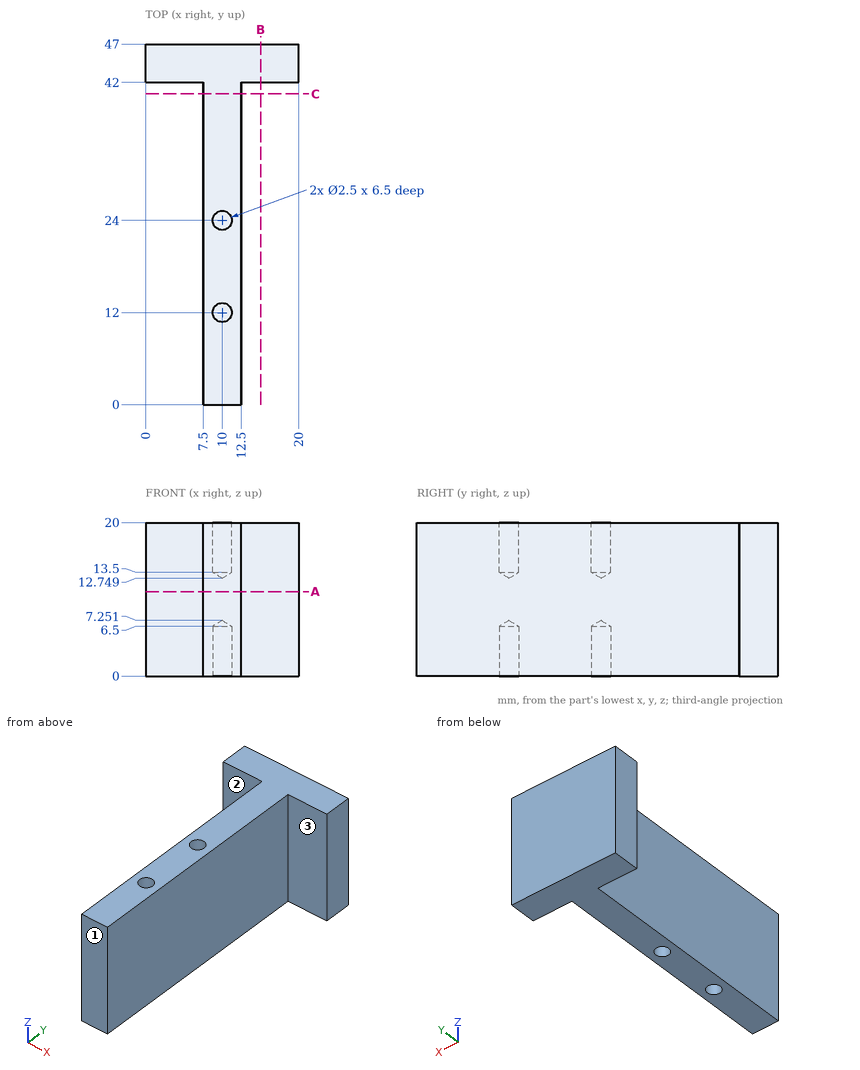
Verification items for this drawing (mm, ordinates from the low corner). A direction names the side the tool comes from. Coordinates: 2 decimals unless noted, no trailing zeros. Loops run counter-clockwise (first coordinate to the right, second up) from the corner with the lowest first, then second, coordinate; pieces in that order, holes last.
Item 1: Access from +Z, -Z, +X, -X, +Y, -Y to the whole of each face (thin tool, end or side, straight path). Record for the marked faces 1, 2 and 3.
Item 2: Thickness scan on line 1 (Y direction, x = 10, z = 15.75); line 2 (X direction, y = 12, z = 3.25); line 3 (Y direction, x = 15.5, z = 12.5). Record the ranges inside material, lowest first.
Item 3: Go/stop test with flat-tipped pins: pin 1 Ø5 at (y, z) = (6.5, 14) entering from +X; pin 2 Ø12 at (y, z) = (18.5, 8) entering from -X; pin 3 Ø4 at (x, z) = (15, 6) entering from -Y. Record where each tip stops, or that it passes through.
Item 4: Sectioned sample at C-C, the plane y = 40.5. Record the boundary of the cut face in (x, z).
Item 5: Sectioned sample at B-B, the plane x = 15. Record the boundary of the cut face in (y, z).
Item 6: Sectioned sample at A-A, the plane z = 11. Record the boundary of the cut face in (x, y).
Check result:
1. face 1: +Z, -Z, +X, -X, -Y
1. face 2: +Z, -Z, -X, -Y
1. face 3: +Z, -Z, +X, -Y
2. line 1: y = 0 to 10.75, 13.25 to 22.75, 25.25 to 47
2. line 2: x = 7.5 to 8.75, 11.25 to 12.5
2. line 3: y = 42 to 47
3. pin 1: stops at x = 12.5
3. pin 2: stops at x = 7.5
3. pin 3: stops at y = 42
4. outline: (7.5, 0) - (12.5, 0) - (12.5, 20) - (7.5, 20) - close
5. outline: (42, 0) - (47, 0) - (47, 20) - (42, 20) - close
6. outline: (0, 42) - (7.5, 42) - (7.5, 0) - (12.5, 0) - (12.5, 42) - (20, 42) - (20, 47) - (0, 47) - close
